Source: CAD feature listing. Evaluate the final solid. Frame: model axes, mm. A direction names the side the tool comes from. Give positions to 0.01 mm unless a question says otherwise; leave off trailing zeros. Write each loop counter-clockwise with the first axis right and the second up, starting at its lowest first coordinate (ties: lowest second). Pieces come first, ordered by that corner, then holes. Notation, with made-up numbers: (65, 77.5) -> (74, 77.5) arc R24 cw to (74, 112.5) -> close; hole circle Ø2 at (-17, 44). An arc over 180 degrees is marked (long way). Write item = value, one per line.
from build123d import *

# Parameters (mm, degrees)
DODANIE_WYCI_GNI_CIE1_DEPTH = 50
ZAOKR_GLENIE1_R             = 50


with BuildPart() as part:
    # Szkic1 → Dodanie-wyciągnięcie1 (new body)
    with BuildSketch(Plane.XY):
        Polygon((-250, -10), (250, -10), (1282.526348129, 365.808856814), (1276.107770084, 383.443755056), (250, 9.971069596), (250, 10), (-250, 10), align=None)
    extrude(amount=DODANIE_WYCI_GNI_CIE1_DEPTH)

    # Zaokrąglenie1
    # the kernel refuses this fillet: 50 mm, written as the material it takes off along each edge
    with BuildSketch(Plane(origin=(250, 10, -4.251619831), x_dir=(0, -1, 0), z_dir=(0, 0, 1))) as zaokr_glenie1_piece_1:
        with BuildLine():
            CenterArc((50, -1.700647932), ZAOKR_GLENIE1_R, 178.05082507, 1.94917493)
            Line((0, -1.700647932), (0, 0))
            Line((0, 0), (0.028930404, 0))
        make_face()
    extrude(amount=58.503239662, mode=Mode.SUBTRACT)
    with BuildSketch(Plane(origin=(250, -10, -22.040872589), x_dir=(-1, 0, 0), z_dir=(0, 0, 1))) as zaokr_glenie1_piece_2:
        with BuildLine():
            CenterArc((ZAOKR_GLENIE1_R * 0.176326980708, -ZAOKR_GLENIE1_R), ZAOKR_GLENIE1_R, 90, 20)
            Line((-ZAOKR_GLENIE1_R * 0.165693162617, -ZAOKR_GLENIE1_R * 0.0603073792141), (0, 0))
            Line((0, 0), (ZAOKR_GLENIE1_R * 0.176326980708, 0))
        make_face()
    extrude(amount=94.081745177, mode=Mode.SUBTRACT)


solid = part.part
1) Material intervals for L1, parallel to Y at x = 53.5, z = 16; L2, parallel to Y at x = 245.5, z = 23, sorted ascending.
Computed:
L1 = -10 to 10
L2 = -9.81 to 10
2) Access query for faces 1 (the flat face through (-8, -10, 25)), 2 (the flat face through (3, 10, 25)). Directions: +Z, -Z, +X, -X, +Y, -Y. A direction counts if a zero-diameter tool reaches every point of the face in a straight line with its end or side. Return the directions, or none.
Computed:
face_1 = +Z, -Z, +X, -X, -Y
face_2 = +Z, -Z, -X, +Y
3) Cut plane A-A (z = 14). Return the cut outline in (x, y), then the cut area to 3 significant figures.
Computed:
outline = (-250, -10) -> (241.18, -10) arc R50 ccw to (258.28, -6.98) -> (1282.53, 365.81) -> (1276.11, 383.44) -> (250, 9.97) arc R50 ccw to (248.3, 10) -> (-250, 10) -> close
area = 30,600 mm²
4) Cut plane B-B (x = 69). Return the cut outline in (y, z), then the cut area to 3 significant figures.
Computed:
outline = (-10, 0) -> (10, 0) -> (10, 50) -> (-10, 50) -> close
area = 1,000 mm²
5) Contact query for a flat-ended pin moving along its axis: pin 1 (5 mm diameter, centred on x = 1077, z = 10.5, fed in from +Y). Output: stop coordinate, or through.
Computed:
pin_1 = 311.88
6) Cut plane C-C (y = 154). Return the cut outline in (x, z), then the cut area to 3 significant figures.
Computed:
outline = (645.72, 0) -> (700.59, 0) -> (700.59, 50) -> (645.72, 50) -> close
area = 2,740 mm²
